Geometry check sheet. Reference: the model listing, model coordinates, mm. Give positions to 0.01 mm unless a question says otherwise; leave off trailing zeros. Order: outer loops, then holes, each group sorted by start corner. A loop starts at its lowest first (then second) coordinate and runs counter-clockwise, first axis right, second up.
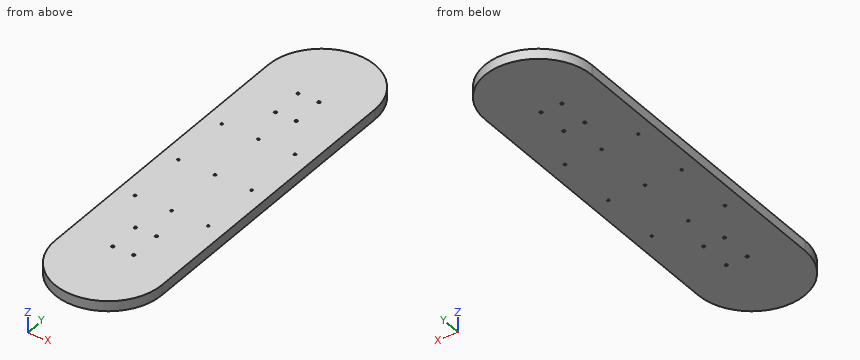
Autodesk Inventor part; units mm, degrees
ref_plane "作業平面1" through (6614.749, 337.2794, 0) normal (0, 0, 1) x (1, 0, 0)
sketch "スケッチ1" plane through (6614.749, 337.2794, 0) normal (0, 0, 1) x (1, 0, 0)
  line L0 (-6509.749, -42.2794) -> (-6509.749, -632.2794)
  line L1 (-6509.749, -632.2794) -> (-6719.749, -632.2794)
  line L2 (-6719.749, -632.2794) -> (-6719.749, -42.2794)
  line L3 (-6719.749, -42.2794) -> (-6509.749, -42.2794)
  arc A0 (-6509.749, -42.2794) -> (-6719.749, -42.2794) centre (-6614.749, -42.2794) ccw
  arc A1 (-6719.749, -632.2794) -> (-6509.749, -632.2794) centre (-6614.749, -632.2794) ccw
  line L4 (-6614.749, -897.2794) -> (-6614.749, 222.7206)
  line L5 (-8036.2537, -337.2794) -> (1179.2797, -337.2794)
  line L6 (-6509.749, -337.2794) -> (-137.2251, -337.2794)
  point P0 (-6614.749, -337.2794)
  dimension "d1" = 210
  dimension "d3" = 105
  dimension "d4" = 590
  dimension "d5" = 105
  dimension "d8" = 295
extrude "押し出し1" add sketch "スケッチ1" along normal blind 20
sketch "スケッチ2" plane through (6614.749, 337.2794, 0) normal (0, 0, -1) x (-1, 0, 0)
  spline S0 degree 3 poles (6630.8363, -557.2765) (6630.8356, -556.4314) (6630.8307, -555.5861) (6630.7821, -551.1548) (6630.6652, -547.5706) (6630.2129, -540.6292) (6629.8924, -537.269) (6629.059, -531.5504) (6628.6277, -529.1809) (6627.5, -524.5004) (6626.8057, -522.1844) (6625.8839, -519.9595) knots -3.785676 -3.785676 -3.785676 -3.785676 -3.532131 -3.532131 -2.4562 -2.4562 -1.444966 -1.444966 -0.722485 -0.722485 0 0 0 0
  spline S1 degree 3 poles (6630.0302, -579.9499) (6630.1435, -578.1819) (6630.247, -576.4134) (6630.4408, -572.7081) (6630.5289, -570.7713) (6630.6019, -568.834) (6630.6759, -566.8669) (6630.7344, -564.8993) (6630.8129, -561.0466) (6630.8346, -559.1616) (6630.8363, -557.2765) knots -2.294162 -2.294162 -2.294162 -2.294162 -1.762693 -1.762693 -1.181069 -1.181069 -1.181069 -0.590534 -0.590534 -0.025021 -0.025021 -0.025021 -0.025021
  spline S2 degree 3 poles (6629.9005, -581.946) (6629.933, -581.4474) (6629.9654, -580.9489) (6629.9979, -580.4504) (6630.0033, -580.367) (6630.0087, -580.2836) (6630.0195, -580.1167) (6630.0249, -580.0333) (6630.0302, -579.9499) knots -0.65131 -0.65131 -0.65131 -0.65131 -0.501438 -0.501438 -0.501438 -0.47636 -0.47636 -0.451282 -0.451282 -0.451282 -0.451282
  ellipse E0 centre (6627.749, -583.7463) end of major axis (6627.749, -580.2108) minor radius 2.5 (6630.249, -583.7463) -> (6629.9005, -581.946) ccw
  line L0 (6630.249, -596.9595) -> (6630.249, -583.7463)
  line L1 (6640.249, -596.9595) -> (6630.249, -596.9595)
  arc A0 (6640.249, -596.9595) -> (6641.749, -595.4595) centre (6640.249, -595.4595) ccw
  line L2 (6641.749, -521.4595) -> (6641.749, -595.4595)
  arc A1 (6641.749, -521.4595) -> (6640.249, -519.9595) centre (6640.249, -521.4595) ccw
  line L3 (6625.8839, -519.9595) -> (6640.249, -519.9595)
  circle A2 centre (6635.249, -591.4595) radius 3
  circle A3 centre (6635.249, -528.4595) radius 3
  circle A4 centre (6594.249, -591.4595) radius 3
  circle A5 centre (6594.249, -528.4595) radius 3
  spline S3 degree 3 poles (6599.4677, -579.9499) (6599.473, -580.0333) (6599.4784, -580.1167) (6599.4892, -580.2836) (6599.4946, -580.367) (6599.5, -580.4504) (6599.5325, -580.9489) (6599.5649, -581.4474) (6599.5974, -581.946) knots -0.050156 -0.050156 -0.050156 -0.050156 -0.025078 -0.025078 0 0 0 0.149872 0.149872 0.149872 0.149872
  spline S4 degree 3 poles (6598.6616, -557.2765) (6598.6633, -559.1539) (6598.6848, -561.0313) (6598.7628, -564.8687) (6598.8208, -566.8287) (6598.8943, -568.7881) (6598.9673, -570.7332) (6599.0556, -572.6776) (6599.25, -576.3981) (6599.3539, -578.1743) (6599.4677, -579.9499) knots -2.319296 -2.319296 -2.319296 -2.319296 -1.756075 -1.756075 -1.167834 -1.167834 -1.167834 -0.583917 -0.583917 -0.050156 -0.050156 -0.050156 -0.050156
  spline S5 degree 3 poles (6603.614, -519.9595) (6602.3019, -523.1265) (6601.4408, -526.4662) (6600.1974, -532.85) (6599.7845, -535.9073) (6599.0649, -543.0901) (6598.8445, -547.2235) (6598.6873, -553.3316) (6598.6634, -555.3041) (6598.6616, -557.2765) knots -3.810629 -3.810629 -3.810629 -3.810629 -2.782212 -2.782212 -1.858006 -1.858006 -0.616716 -0.616716 -0.024978 -0.024978 -0.024978 -0.024978
  line L4 (6589.249, -519.9595) -> (6603.614, -519.9595)
  arc A6 (6589.249, -519.9595) -> (6587.749, -521.4595) centre (6589.249, -521.4595) ccw
  line L5 (6587.749, -595.4595) -> (6587.749, -521.4595)
  arc A7 (6587.749, -595.4595) -> (6589.249, -596.9595) centre (6589.249, -595.4595) ccw
  line L6 (6599.249, -596.9595) -> (6589.249, -596.9595)
  line L7 (6599.249, -583.7463) -> (6599.249, -596.9595)
  ellipse E1 centre (6601.749, -583.7463) end of major axis (6601.749, -580.2108) minor radius 2.5 (6599.5974, -581.946) -> (6599.249, -583.7463) ccw
  spline S6 degree 3 poles (6630.8363, -107.2765) (6630.8356, -106.4314) (6630.8307, -105.5861) (6630.7821, -101.1548) (6630.6652, -97.5706) (6630.2129, -90.6292) (6629.8924, -87.269) (6629.059, -81.5504) (6628.6277, -79.1809) (6627.5, -74.5004) (6626.8057, -72.1844) (6625.8839, -69.9595) knots -3.785676 -3.785676 -3.785676 -3.785676 -3.532131 -3.532131 -2.4562 -2.4562 -1.444966 -1.444966 -0.722485 -0.722485 0 0 0 0
  spline S7 degree 3 poles (6630.0302, -129.9499) (6630.1435, -128.1819) (6630.247, -126.4134) (6630.4408, -122.7081) (6630.5289, -120.7713) (6630.6019, -118.834) (6630.6759, -116.8669) (6630.7344, -114.8993) (6630.8129, -111.0466) (6630.8346, -109.1616) (6630.8363, -107.2765) knots -2.294162 -2.294162 -2.294162 -2.294162 -1.762693 -1.762693 -1.181069 -1.181069 -1.181069 -0.590534 -0.590534 -0.025021 -0.025021 -0.025021 -0.025021
  spline S8 degree 3 poles (6629.9005, -131.946) (6629.933, -131.4474) (6629.9654, -130.9489) (6629.9979, -130.4504) (6630.0033, -130.367) (6630.0087, -130.2836) (6630.0195, -130.1167) (6630.0249, -130.0333) (6630.0302, -129.9499) knots -0.65131 -0.65131 -0.65131 -0.65131 -0.501438 -0.501438 -0.501438 -0.47636 -0.47636 -0.451282 -0.451282 -0.451282 -0.451282
  ellipse E2 centre (6627.749, -133.7463) end of major axis (6627.749, -130.2108) minor radius 2.5 (6630.249, -133.7463) -> (6629.9005, -131.946) ccw
  line L8 (6630.249, -146.9595) -> (6630.249, -133.7463)
  line L9 (6640.249, -146.9595) -> (6630.249, -146.9595)
  arc A8 (6640.249, -146.9595) -> (6641.749, -145.4595) centre (6640.249, -145.4595) ccw
  line L10 (6641.749, -71.4595) -> (6641.749, -145.4595)
  arc A9 (6641.749, -71.4595) -> (6640.249, -69.9595) centre (6640.249, -71.4595) ccw
  line L11 (6625.8839, -69.9595) -> (6640.249, -69.9595)
  circle A10 centre (6635.249, -141.4595) radius 3
  circle A11 centre (6635.249, -78.4595) radius 3
  circle A12 centre (6594.249, -141.4595) radius 3
  circle A13 centre (6594.249, -78.4595) radius 3
  spline S9 degree 3 poles (6599.4677, -129.9499) (6599.473, -130.0333) (6599.4784, -130.1167) (6599.4892, -130.2836) (6599.4946, -130.367) (6599.5, -130.4504) (6599.5325, -130.9489) (6599.5649, -131.4474) (6599.5974, -131.946) knots -0.050156 -0.050156 -0.050156 -0.050156 -0.025078 -0.025078 0 0 0 0.149872 0.149872 0.149872 0.149872
  spline S10 degree 3 poles (6598.6616, -107.2765) (6598.6633, -109.1539) (6598.6848, -111.0313) (6598.7628, -114.8687) (6598.8208, -116.8287) (6598.8943, -118.7881) (6598.9673, -120.7332) (6599.0556, -122.6776) (6599.25, -126.3981) (6599.3539, -128.1743) (6599.4677, -129.9499) knots -2.319296 -2.319296 -2.319296 -2.319296 -1.756075 -1.756075 -1.167834 -1.167834 -1.167834 -0.583917 -0.583917 -0.050156 -0.050156 -0.050156 -0.050156
  spline S11 degree 3 poles (6603.614, -69.9595) (6602.3019, -73.1265) (6601.4408, -76.4662) (6600.1974, -82.85) (6599.7845, -85.9073) (6599.0649, -93.0901) (6598.8445, -97.2235) (6598.6873, -103.3316) (6598.6634, -105.3041) (6598.6616, -107.2765) knots -3.810629 -3.810629 -3.810629 -3.810629 -2.782212 -2.782212 -1.858006 -1.858006 -0.616716 -0.616716 -0.024978 -0.024978 -0.024978 -0.024978
  line L12 (6589.249, -69.9595) -> (6603.614, -69.9595)
  arc A14 (6589.249, -69.9595) -> (6587.749, -71.4595) centre (6589.249, -71.4595) ccw
  line L13 (6587.749, -145.4595) -> (6587.749, -71.4595)
  arc A15 (6587.749, -145.4595) -> (6589.249, -146.9595) centre (6589.249, -145.4595) ccw
  line L14 (6599.249, -146.9595) -> (6589.249, -146.9595)
  line L15 (6599.249, -133.7463) -> (6599.249, -146.9595)
  ellipse E3 centre (6601.749, -133.7463) end of major axis (6601.749, -130.2108) minor radius 2.5 (6599.5974, -131.946) -> (6599.249, -133.7463) ccw
  point P0 (6614.749, -337.2794)
hole "穴1" at (-20.5, -191.1802, 0) at (20.5, -191.1802, 0) at (20.5, -254.1802, 0) at (-20.5, -254.1802, 0) at (-20.5, 258.8198, 0) at (20.5, 258.8198, 0) at (-20.5, 195.8198, 0) at (20.5, 195.8198, 0) direction (0, 0, 1) diameter 5.5 end through all
sketch "スケッチ4" plane through (0, 0, 0) normal (0, 0, 1) x (1, 0, 0)
  circle A0 centre (-20.5, 195.8198) radius 2.75
  circle A1 centre (-20.5, 258.8198) radius 2.75
  circle A2 centre (20.5, -254.1802) radius 2.75
  circle A3 centre (-20.5, -191.1802) radius 2.75
  circle A4 centre (20.5, -191.1802) radius 2.75
  circle A5 centre (-20.5, -254.1802) radius 2.75
  circle A6 centre (20.5, 258.8198) radius 2.75
  circle A7 centre (20.5, 195.8198) radius 2.75
  arc A8 (105, 295) -> (-105, 295) centre (0, 295) ccw
  line L0 (-105, 295) -> (-105, -295)
  arc A9 (-105, -295) -> (105, -295) centre (0, -295) ccw
  line L1 (105, -295) -> (105, 295)
  line L2 (65, -50) -> (65, 50)
  line L3 (30, 50) -> (30, -50)
  line L4 (30, -50) -> (65, 50) construction
  line L5 (65, -50) -> (30, 50) construction
  arc A10 (30, -50) -> (65, -50) centre (47.5, -40.3175) ccw
  line L6 (-147, 0) -> (147, 0)
  arc A11 (65, 50) -> (30, 50) centre (47.5, 40.3175) ccw
  point P0 (0, 0)
  point P1 (47.5, 0)
  dimension "d16" = 35
  dimension "d17" = 100
  dimension "d18" = 40
  dimension "d19" = 20
  dimension "d20" = 20
extrude "押し出し2" [suppressed]
sketch "スケッチ6" plane through (6614.749, 337.2794, 0) normal (0, 0, -1) x (-1, 0, 0)
  line L0 (6467.749, -337.2794) -> (6761.749, -337.2794)
  line L1 (6614.749, -897.2794) -> (6614.749, 222.7206)
  point P0 (6614.749, -337.2794)
  point P1 (6614.749, -337.2794)
  point P2 (6542.749, -337.2794)
  point P3 (6542.749, -457.2794)
  point P4 (6614.749, -457.2794)
  point P5 (6614.749, -337.2794)
  point P6 (6542.749, -217.2794)
  point P7 (6614.749, -217.2794)
  point P8 (6686.749, -337.2794)
  point P9 (6686.749, -457.2794)
  point P10 (6686.749, -217.2794)
  dimension "d23" = 120
  dimension "d24" = 72
  dimension "d25" = 72
hole "穴2" at (0, 0, 0) at (72, 0, 0) at (72, -120, 0) at (0, -120, 0) at (0, 120, 0) at (72, 120, 0) at (-72, -120, 0) at (-72, 0, 0) at (-72, 120, 0) direction (0, 0, 1) diameter 4.5 end through all
equation "\"d5\" = 0.5 * d1"
equation "\"d8\" = 0.5 * d4"
equation "\"d20\" = d19"
properties part number "board" material "木材(サクラ)"
Item 1: Sectioned sample at A-A (z = 5.25). Give the number of separate pieces and of enclosed holes in the cut face, and give its area (3 significant figures).
Reported:
separate pieces: 1
enclosed holes: 17
area: 158,000 mm2
Item 2: Sectioned sample at C-C (x = -55). Enter the section's corners in (y, z), and give its area (3 significant figures).
Reported:
outline: (-384.44, 0) - (384.44, 0) - (384.44, 20) - (-384.44, 20) - close
area: 15,400 mm2
Item 3: Gauge pin test, flat ends, axial feed: pin 1 (6 mm diameter, centred on x = -59.5, z = 8, fed in from -Y); pin 2 (7 mm diameter, centred on x = 0, y = 0, fed in from -Z); pin 3 (3.5 mm diameter, centred on x = 0, y = -120, fed in from -Z); pin 4 (3 mm diameter, centred on x = -46.5, z = 11, fed in from +Y). Record the tip position at first contact, or that the pin passes through.
Reported:
pin 1: stops at y = -383.5
pin 2: stops at z = 0
pin 3: passes through
pin 4: stops at y = 389.87
Item 4: Scan lines: L1, parallel to X at y = 120, z = 9; L2, parallel to Y at x = 0, z = 13.5; L3, parallel to Y at x = -72, z = 11. Record each from-to range of solid material in increasing order.
Reported:
L1: x = -105 to -74.25, -69.75 to -2.25, 2.25 to 69.75, 74.25 to 105
L2: y = -400 to -122.25, -117.75 to -2.25, 2.25 to 117.75, 122.25 to 400
L3: y = -371.43 to -122.25, -117.75 to -2.25, 2.25 to 117.75, 122.25 to 371.43
Item 5: Sectioned sample at B-B (x = -85.5). Enter the section's corners in (y, z).
Reported:
outline: (-355.95, 0) - (355.95, 0) - (355.95, 20) - (-355.95, 20) - close
